CAD build for the part. Positions are in the model's coordinates, mm. A direction names the side the tool comes from. Give positions to 0.01 mm unless a question says otherwise; leave off trailing zeros. Write each loop counter-clockwise with the first axis right and the second up, starting at its lowest first coordinate (ties: lowest second). Pieces come first, ordered by that corner, then holes. Notation, with made-up numbers: (76.25, 4.25) - (96.25, 4.25) arc R32 ccw to (96.25, 40.25) - close; hole circle Ø9 at (37, 0). An arc over 180 degrees is marked (long way). Answer as a JSON object with one key per item and string values.
Autodesk Inventor part; units mm, degrees
ref_plane "Work Plane2" through (0, 0, -3.175) normal (0, 0, 1) x (1, 0, 0)
ref_plane "YZ Plane" through (0, 0, 0) normal (1, 0, 0) x (0, 1, 0)
ref_plane "XZ Plane" through (0, 0, 0) normal (0, 1, 0) x (-1, 0, 0)
sketch "Sketch1" plane through (0, 0, 0) normal (0, 0, 1) x (1, 0, 0)
  line L0 (-31.75, 110.3249) -> (31.75, 110.3249)
  line L1 (31.75, 110.3249) -> (31.75, 8.7249)
  line L2 (-31.75, 8.7249) -> (-31.75, 110.3249)
  line L3 (-31.75, 8.7249) -> (-19.05, 8.7249)
  line L4 (31.75, 8.7249) -> (19.05, 8.7249)
  line L5 (-19.05, 8.7249) -> (-19.05, 21.4249)
  line L6 (19.05, 8.7249) -> (19.05, 21.4249)
  arc A0 (19.05, 21.4249) -> (-19.05, 21.4249) centre (0, 21.4249) ccw
  point P0 (0, 0)
  dimension "d0" = 63.5
  dimension "d1" = 31.75
  dimension "d2" = 101.6
  dimension "d3" = 110.3249
  dimension "d4" = 12.7
  dimension "d5" = 12.7
  dimension "d46" = 101.6
  dimension "d52" = 12.7
  dimension "d53" = 12.7
extrude "Extrusion1" add sketch "Sketch1" against normal blind 6.35
sketch "Sketch2" plane through (31.75, 8.7249, 0) normal (1, 0, 0) x (0, 0, -1)
  line L0 (6.35, 0) -> (6.35, 101.6)
  line L1 (0, 101.6) -> (6.35, 101.6)
  line L2 (0, 101.6) -> (0, 0)
  line L3 (0, 0) -> (6.35, 0)
  point P0 (0, -8.7249)
  point P1 (3.175, 3.175)
  point P2 (3.175, 88.9)
  point P3 (3.175, 50.8)
  dimension "d22" = 12.7
  dimension "d23" = 3.175
  dimension "d24" = 3.175
  dimension "d25" = 3.175
  dimension "d54" = 50.8
  dimension "d55" = 3.175
hole "Hole2" at (31.75, 11.8999, -3.175) at (31.75, 97.6249, -3.175) at (31.75, 59.5249, -3.175) direction (-1, 0, 0) diameter 3.175 depth 9.525 tip angle 118
sketch "Sketch3" plane through (-31.75, 8.7249, 0) normal (-1, 0, 0) x (0, 0, 1)
  line L0 (0, 0) -> (-6.35, 0)
  line L1 (0, 0) -> (0, 101.6)
  line L2 (0, 101.6) -> (-6.35, 101.6)
  line L3 (-6.35, 101.6) -> (-6.35, 0)
  point P0 (0, -8.7249)
  point P1 (-3.175, 88.9)
  point P2 (-3.175, 3.175)
  point P3 (-3.175, 50.8)
  dimension "d33" = 3.175
  dimension "d34" = 12.7
  dimension "d35" = 3.175
  dimension "d36" = 3.175
  dimension "d56" = 50.8
  dimension "d57" = 3.175
hole "Hole3" at (-31.75, 97.6249, -3.175) at (-31.75, 11.8999, -3.175) at (-31.75, 59.5249, -3.175) direction (1, 0, 0) diameter 3.175 depth 9.525 tip angle 118
sketch "Sketch5" plane through (-31.75, 110.3249, 0) normal (0, 1, 0) x (1, 0, 0)
  line L0 (0, 0) -> (0, 6.35)
  line L1 (0, 0) -> (63.5, 0)
  line L2 (63.5, 0) -> (63.5, 6.35)
  point P0 (31.75, 0)
  point P1 (3.175, 3.175)
  point P2 (60.325, 3.175)
  dimension "d78" = 3.175
  dimension "d79" = 3.175
  dimension "d80" = 3.175
hole "Hole4" at (-28.575, 110.3249, -3.175) at (28.575, 110.3249, -3.175) direction (0, -1, 0) diameter 3.175 depth 9.525 tip angle 118
ref_plane "Work Plane2" through (0, 0, -3.175) normal (0, 0, 1) x (1, 0, 0)
sketch "Sketch6" plane through (0, 0, -3.175) normal (0, 0, 1) x (1, 0, 0)
  arc A0 (25.4, 21.4249) -> (-25.4, 21.4249) centre (0, 21.4249) ccw
  line L0 (-31.75, 110.3249) -> (-31.75, 8.7249)
  line L1 (31.75, 110.3249) -> (-31.75, 110.3249)
  line L2 (31.75, 8.7249) -> (31.75, 110.3249)
  line L3 (19.05, 8.7249) -> (31.75, 8.7249)
  arc A1 (19.05, 21.4249) -> (-19.05, 21.4249) centre (0, 21.4249) ccw
  line L4 (19.05, 21.4249) -> (19.05, 8.7249)
  line L5 (-19.05, 8.7249) -> (-19.05, 21.4249)
  line L6 (-31.75, 8.7249) -> (-19.05, 8.7249)
  line L7 (-25.4, 21.4249) -> (-25.4, 103.9749)
  line L8 (-25.4, 103.9749) -> (25.4, 103.9749)
  line L9 (25.4, 103.9749) -> (25.4, 21.4249)
  line L10 (25.4, 103.9749) -> (-25.4, 53.1749) construction
  line L11 (-25.4, 103.9749) -> (25.4, 53.1749) construction
  line L12 (-25.4, 99.4848) -> (-4.4901, 78.5749)
  line L13 (-4.4901, 78.5749) -> (-25.4, 57.665)
  line L14 (-20.9099, 103.9749) -> (0, 83.065)
  line L15 (0, 83.065) -> (20.9099, 103.9749)
  line L16 (25.4, 99.4848) -> (4.4901, 78.5749)
  line L17 (4.4901, 78.5749) -> (25.4, 57.665)
  line L18 (-25.4, 48.6848) -> (0, 74.0848)
  line L19 (0, 74.0848) -> (25.4, 48.6848)
  arc A2 (-25.4, 65.3302) -> (-19.9799, 63.0851) centre (-22.225, 65.3302) ccw
  arc A3 (-19.9799, 94.0647) -> (-25.4, 91.8196) centre (-22.225, 91.8196) ccw
  arc A4 (25.4, 91.8196) -> (19.9799, 94.0647) centre (22.225, 91.8196) ccw
  arc A5 (19.9799, 63.0851) -> (25.4, 65.3302) centre (22.225, 65.3302) ccw
  point P0 (0, 0)
  dimension "d99" = 25.4
  dimension "d100" = 6.35
  dimension "d101" = 6.35
  dimension "d102" = 6.35
  dimension "d103" = 45
  dimension "d104" = 6.35
  dimension "d105" = 3.175
  dimension "d106" = 3.175
  dimension "d108" = 6.35
  dimension "d109" = 3.175
  dimension "d110" = 6.35
  dimension "d111" = 3.175
  dimension "d112" = 6.35
  dimension "d113" = 3.175
  dimension "d114" = 3.175
  dimension "d115" = 3.175
  dimension "d116" = 3.175
extrude "Extrusion5" cut sketch "Sketch6" along normal mid plane 25.4 contours A0 L7 L18 L19 L9 | A5 L17 L16 A4 L9 | L7 A3 L12 L13 A2 | L15 L14 L8
fillet "Fillet3" radius 3.175 10 edges at (-25.4, 21.4249, -3.175) (25.4, 21.4249, -3.175) (25.4, 48.6848, -3.175) (0, 74.0848, -3.175) (-25.4, 48.6848, -3.175) (-4.4901, 78.5749, -3.175) (4.4901, 78.5749, -3.175) (0, 83.065, -3.175) (-20.9099, 103.9749, -3.175) (20.9099, 103.9749, -3.175)
equation "\"d105\" = 0.5 * d104"
equation "\"d106\" = d105"
equation "\"d109\" = d105"
equation "\"d110\" = d108"
equation "\"d111\" = d105"
equation "\"d112\" = d104"
properties part number "lower box front plate2"
Item 1: Cut at B-B (y = 31). Give the cut face in (x, z), and give its area (3 significant figures).
Entries:
{"outline": "(-31.75, -6.35) - (-16.47, -6.35) - (-16.47, 0) - (-31.75, 0) - close; (16.47, -6.35) - (31.75, -6.35) - (31.75, 0) - (16.47, 0) - close", "area": "194 mm2"}
Item 2: Which spindle directions (+Z, -Z, +X, -X, +Y, -Y) get a long thin tool onto all of the face, cutting with end or side? Do faces 3 (the flat face through (25, 8.725, -3)), 4 (the cylindrical face through (23.49, 62.42, -3.22)), 5 (the cylindrical face through (26.92, 12.87, -1.92)), 6 (the cylindrical face through (-26.921, 99.175, -3.519)). Say none if no direction does.
Entries:
{"face 3": "+Z, -Z, +X, -X, -Y", "face 4": "+Z, -Z", "face 5": "+X", "face 6": "-X"}
Item 3: Mould opens along Z. For faces 1 (the conical face through (-21.437, 97.38, -3.048)), 2 (the cylindrical face through (25.165, 48.569, -3.131)) say: +Z half, -Z half, draft (parallel to the pull), parting line (faces both ways), or undercut.
Entries:
{"face 1": "undercut", "face 2": "draft"}
Item 4: Cut at A-A (x = 0). Give the cut face in (y, z), and give its area (3 significant figures).
Entries:
{"outline": "(40.47, -6.35) - (46.82, -6.35) - (46.82, 0) - (40.47, 0) - close; (72.77, -6.35) - (84.38, -6.35) - (84.38, 0) - (72.77, 0) - close; (103.97, -6.35) - (110.32, -6.35) - (110.32, 0) - (103.97, 0) - close", "area": "154 mm2"}
Item 5: Probe line 1 (Y direction, x = -5, z = -5) (3 decimals); line 2 (Y direction, x = 27.5, z = -3); line 3 (X direction, y = 88.5, z = -5.5) (3 decimals). List the from-to ranges inside material, lowest first. Write a range as from..to.
Entries:
{"line 1": "39.807..46.328, 69.085..88.065, 103.975..110.325", "line 2": "8.72..10.32, 13.48..57.95, 61.1..96.05, 99.2..100.5", "line 3": "-31.75..-25.4, -14.415..-5.435, 5.435..14.415, 25.4..31.75"}
Item 6: Flat gauge pins, fed straight in: P1, Ø3, axis at y = 11.9, z = -3.18, coming from the -X side; P2, Ø2, axis at x = 14.5, z = -5.5, coming from the -Y side; P3, Ø2.5, axis at y = 59.52, z = -3.18, coming from the -X side; P4, Ø10, axis at x = 22.5, y = 80, coming from the +Z side. Where does each tip first touch, or does it go through?
Entries:
{"P1": "x = -22.18", "P2": "y = 32.5", "P3": "x = -22.03", "P4": "z = 0"}
Item 7: Cut at C-C (y = 67.5). Give the cut face in (x, z) (3 decimals).
Entries:
{"outline": "(-31.75, -6.35) - (-25.4, -6.35) - (-25.4, 0) - (-31.75, 0) - close; (-15.565, -6.35) - (-6.585, -6.35) - (-6.585, 0) - (-15.565, 0) - close; (6.585, -6.35) - (15.565, -6.35) - (15.565, 0) - (6.585, 0) - close; (25.4, -6.35) - (31.75, -6.35) - (31.75, 0) - (25.4, 0) - close"}
